Here's how the part is built. I have some questions about the finished solid (model axes, mm). Round coordinates to 2 decimals unless told otherwise and drop trailing zeros. Loops run counter-clockwise (first coordinate to the right, second up) from the corner with the lowest first, then second, coordinate; pieces in that order, holes last. Notation, with made-up numbers: M 11.25,63 L 26.25,63 A27 cw 26.25,95 Z; hole C -32.5,-30 d4. An arc over 180 degrees is marked long. Answer as a JSON object with one key per item and string values.
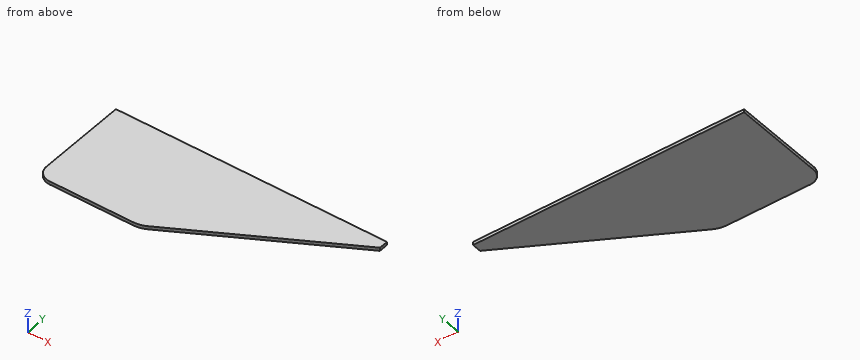
from build123d import *

# Parameters (mm, degrees)
BOSS_EXTRUDE1_DEPTH = 0.79375
FILLET1_R           = 6.35
FILLET2_R           = 12.7


with BuildPart() as part:
    # Sketch1 → Boss-Extrude1 (new, symmetric)
    with BuildSketch(Plane.XY):
        Polygon((0, 0), (-133.35, 0), (-133.35, -50.8), (-82.55, -50.8), (0, -4.5), align=None)
    extrude(amount=BOSS_EXTRUDE1_DEPTH, both=True)

    # Fillet1
    fillet1_edges = [part.edges().sort_by_distance(p)[0] for p in [
        (-133.35, -50.8, 0),
    ]]
    fillet(fillet1_edges, radius=FILLET1_R)

    # Fillet2
    fillet2_edges = [part.edges().sort_by_distance(p)[0] for p in [
        (-82.55, -50.8, 0),
    ]]
    fillet(fillet2_edges, radius=FILLET2_R)


solid = part.part
Item 1: If I drill on L1, parallel to X at y = -30.5, z = 0.15; L2, parallel to Y at x = -66.5, z = 0.45; L3, parallel to Y at x = -55, z = -0.6, over which ranges is the centre line in solid material (lowest first)? Write a range as from..to.
Solution:
{"L1": "x = -133.35..-46.36", "L2": "y = -41.8..0", "L3": "y = -35.35..0"}
Item 2: I want a section at A-A on z = 0. List the corners of the cut face in (x, y) for me, plus the area to 3 significant figures.
Solution:
{"outline": "M -133.35,-44.45 A6.35 ccw -127,-50.8 L -85.87,-50.8 A12.7 ccw -79.66,-49.18 L 0,-4.5 L 0,0 L -133.35,0 Z", "area": "4,850 mm2"}
Item 3: I want a section at C-C on x = -55. List the corners of the cut face in (y, z) for me, plus the area to 3 significant figures.
Solution:
{"outline": "M -35.35,-0.79 L 0,-0.79 L 0,0.79 L -35.35,0.79 Z", "area": "56.1 mm2"}
Item 4: I want a section at B-B on y = -10. List the corners of the cut face in (x, z) for me.
Solution:
{"outline": "M -133.35,-0.79 L -9.81,-0.79 L -9.81,0.79 L -133.35,0.79 Z"}
